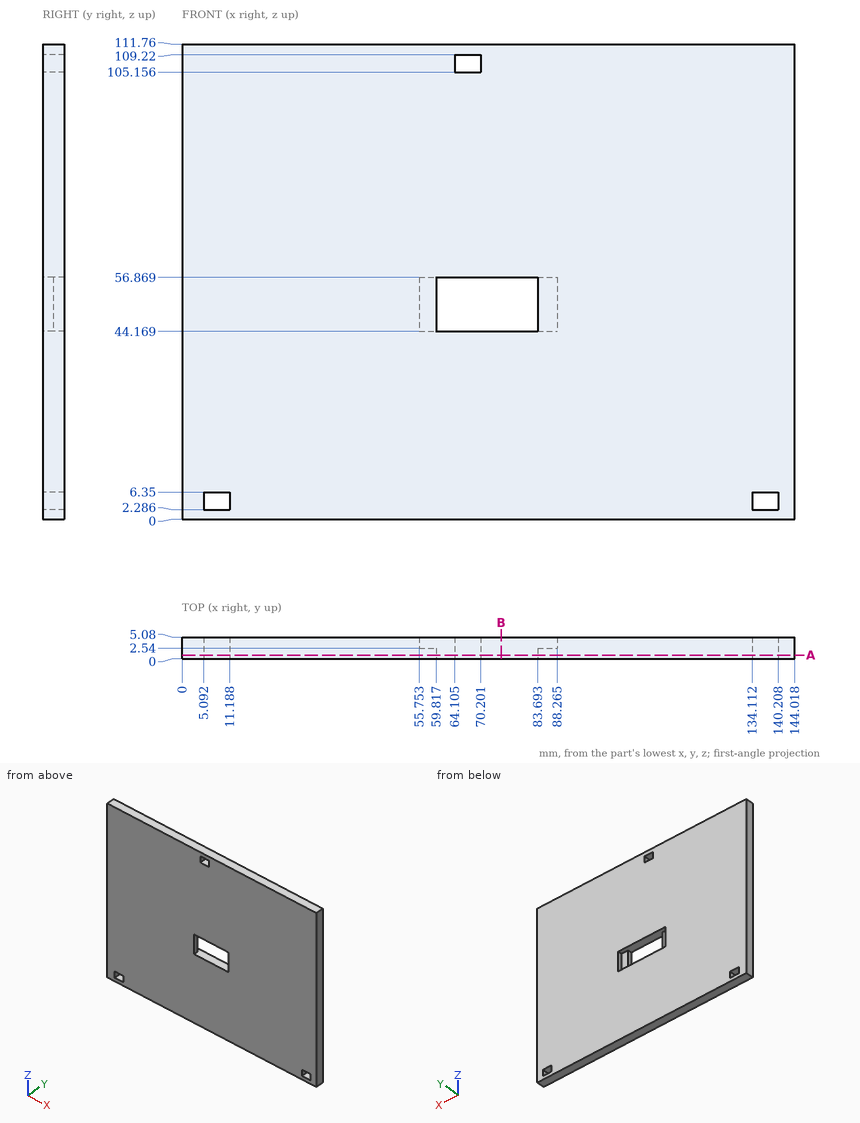
Verification items for this drawing (mm, ordinates from the low corner). Round coordinates to 2 decimals unless told otherwise and drop trailing zeros. Write each loop counter-clockwise with the first axis right and the second up, starting at its lowest first coordinate (ties: lowest second). Pieces come first, ordered by that corner, then holes. Notation, with made-up numbers: (-1.5, -3.5) - (2.5, -3.5) arc R7 ccw to (2.5, 7.5) - close; hole circle Ø3 at (82.5, 22.25). An arc over 180 degrees is marked (long way). One line per item, written item: value.
1. Cross-section at A-A on y = 0.85. Give the number of separate pieces and of enclosed holes in the cut face, and give its area (3 significant figures).
The answers:
separate pieces: 1
enclosed holes: 4
area: 15,700 mm^2
2. Depth check by flat-ended pin: pin 1 Ø1.2 at (x, z) = (57, 52) entering from +Y; pin 2 Ø1 at (x, z) = (103.5, 33) entering from -Y. Enter the tip coordinate at first touch or a pass-through.
The answers:
pin 1: stops at y = 2.54
pin 2: stops at y = 0
3. Cross-section at B-B on x = 75. Record the boundary of the cut face in (y, z), and give its area (3 significant figures).
The answers:
outline: (0, 0) - (5.08, 0) - (5.08, 44.17) - (0, 44.17) - close; (0, 56.87) - (5.08, 56.87) - (5.08, 111.76) - (0, 111.76) - close
area: 503 mm^2
4. Scan lines: L1, parallel to Z at x = 67, y = 0.3 (1 decimal); L2, parallel to Z at x = 72.5, y = 2.25; L3, parallel to X at y = 4.5, z = 49 (1 decimal). Record each from-to range of solid material in increasing order.
The answers:
L1: z = 0 to 44.2, 56.9 to 105.2, 109.2 to 111.8
L2: z = 0 to 44.17, 56.87 to 111.76
L3: x = 0 to 55.8, 88.3 to 144
